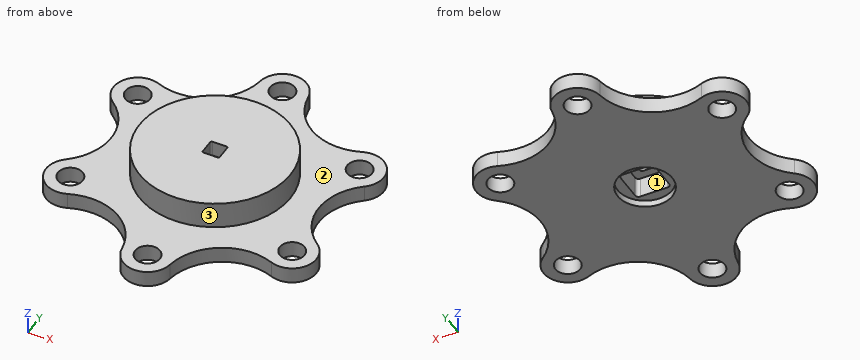
```python
from build123d import *

# Parameters (mm, degrees)
SKETCH1_R           = 2.3
BOSS_EXTRUDE1_DEPTH = 3
SKETCH2_R           = 14
BOSS_EXTRUDE2_DEPTH = 5
CUT_EXTRUDE1_REACH  = 40.688
SKETCH3_W           = 3.175
SKETCH3_H           = 3.175
SKETCH3_3_R         = 5.08
SKETCH3_3_W         = 6.35
SKETCH3_3_H         = 6.35
SKETCH3_3_W_2       = 3.175
SKETCH3_3_H_2       = 3.175
CUT_EXTRUDE2_DEPTH  = 1.27
CUT_EXTRUDE3_START  = -1.27
SKETCH3_4_W         = 6.35
SKETCH3_4_H         = 6.35
SKETCH3_4_W_2       = 3.175
SKETCH3_4_H_2       = 3.175
CUT_EXTRUDE3_DEPTH  = 3.81
FILLET1_R           = 0.254
FILLET2_R           = 0.635


with BuildPart() as part:
    # Sketch1 → Boss-Extrude1 (new body)
    with BuildSketch(Plane.XY):
        with BuildLine():
            ThreePointArc((4.456432387, 24.437168219), (-4.5e-08, 28.3125), (-4.456432399, 24.43716813))
            ThreePointArc((-4.456432399, 24.43716813), (-9.656250022, 16.725115598), (-18.934992245, 16.077967752))
            ThreePointArc((-18.934992245, 16.077967752), (-24.519343502, 14.156251286), (-23.391426978, 8.359202257))
            ThreePointArc((-23.391426978, 8.359202257), (-19.3125, 3.465e-06), (-23.391421517, -8.359197993))
            ThreePointArc((-23.391421517, -8.359197993), (-24.519344633, -14.156249327), (-18.934990017, -16.077966851))
            ThreePointArc((-18.934990017, -16.077966851), (-9.65625113, -16.725114958), (-4.456433088, -24.437163215))
            ThreePointArc((-4.456433088, -24.437163215), (-2.557e-06, -28.3125), (4.456432378, -24.437168281))
            ThreePointArc((4.456432378, -24.437168281), (9.656248045, -16.725116739), (18.934988153, -16.077966097))
            ThreePointArc((18.934988153, -16.077966097), (24.519343112, -14.156251962), (23.391424728, -8.3592005))
            ThreePointArc((23.391424728, -8.3592005), (19.3125, 1.013e-06), (23.391426325, 8.359201747))
            ThreePointArc((23.391426325, 8.359201747), (24.519343744, 14.156250867), (18.934992375, 16.077967805))
            ThreePointArc((18.934992375, 16.077967805), (9.656250044, 16.725115585), (4.456432387, 24.437168219))
        make_face()
        with Locations((0, 23.8125)):
            Circle(SKETCH1_R, mode=Mode.SUBTRACT)
        with Locations((20.622229928, 11.90625)):
            Circle(SKETCH1_R, mode=Mode.SUBTRACT)
        with Locations((-20.622229928, 11.90625)):
            Circle(SKETCH1_R, mode=Mode.SUBTRACT)
        with Locations((20.622229928, -11.90625)):
            Circle(SKETCH1_R, mode=Mode.SUBTRACT)
        with Locations((-20.622229928, -11.90625)):
            Circle(SKETCH1_R, mode=Mode.SUBTRACT)
        with Locations((0, -23.8125)):
            Circle(SKETCH1_R, mode=Mode.SUBTRACT)
    extrude(amount=BOSS_EXTRUDE1_DEPTH)

    # Sketch2 → Boss-Extrude2 (add)
    with BuildSketch(Plane.XY.offset(3)):
        Circle(SKETCH2_R)
    extrude(amount=BOSS_EXTRUDE2_DEPTH)

    # Sketch3 → Cut-Extrude1 (cut, up to next)
    with BuildSketch(Plane(origin=(0, 0, 0), x_dir=(-1, 0, 0), z_dir=(0, 0, -1)), mode=Mode.PRIVATE) as cut_extrude1_sk1:
        Rectangle(SKETCH3_W, SKETCH3_H)
    cut_extrude1_tool1 = extrude(cut_extrude1_sk1.sketch, amount=-CUT_EXTRUDE1_REACH, mode=Mode.PRIVATE) & part.part
    add(cut_extrude1_tool1.solids().sort_by_distance((0, 0, 0))[0], mode=Mode.SUBTRACT)

    # Sketch3<3> → Cut-Extrude2 (cut)
    # profile 1 of 3: a face of its own
    with BuildSketch(Plane(origin=(0, 0, 0), x_dir=(-1, 0, 0), z_dir=(0, 0, -1))):
        Circle(SKETCH3_3_R)
        Rectangle(SKETCH3_3_W, SKETCH3_3_H, mode=Mode.SUBTRACT)
    # profile 2 of 3: a face of its own
    with BuildSketch(Plane(origin=(0, 0, 0), x_dir=(-1, 0, 0), z_dir=(0, 0, -1))):
        Rectangle(SKETCH3_3_W, SKETCH3_3_H)
        Rectangle(SKETCH3_3_W_2, SKETCH3_3_H_2, mode=Mode.SUBTRACT)
    # profile 3 of 3: a face of its own
    with BuildSketch(Plane(origin=(0, 0, 0), x_dir=(-1, 0, 0), z_dir=(0, 0, -1))):
        Rectangle(SKETCH3_3_W_2, SKETCH3_3_H_2)
    extrude(amount=-CUT_EXTRUDE2_DEPTH, mode=Mode.SUBTRACT)

    # Sketch3<4> → Cut-Extrude3 (cut)
    with BuildSketch(Plane(origin=(0, 0, 0), x_dir=(-1, 0, 0), z_dir=(0, 0, -1)).offset(CUT_EXTRUDE3_START)):
        Rectangle(SKETCH3_4_W, SKETCH3_4_H)
        Rectangle(SKETCH3_4_W_2, SKETCH3_4_H_2, mode=Mode.SUBTRACT)
    extrude(amount=-CUT_EXTRUDE3_DEPTH, mode=Mode.SUBTRACT)

    # Fillet1
    fillet1_edges = [part.edges().sort_by_distance(p)[0] for p in [
        (-1.5875, -1.5875, 6.54),
        (1.5875, -1.5875, 6.54),
        (1.5875, 1.5875, 6.54),
        (-1.5875, 1.5875, 6.54),
    ]]
    fillet(fillet1_edges, radius=FILLET1_R)

    # Fillet2
    fillet2_edges = [part.edges().sort_by_distance(p)[0] for p in [
        (3.175, -3.175, 3.175),
        (3.175, 3.175, 3.175),
        (-3.175, 3.175, 3.175),
        (-3.175, -3.175, 3.175),
    ]]
    fillet(fillet2_edges, radius=FILLET2_R)


solid = part.part
```
CAD build for the part. Positions are in the model's coordinates, mm. Face numbers are marked on the shaded views. Coordinates: 2 decimals unless noted, no trailing zeros. Order: outer loops, then holes, each group sorted by start corner. A loop starts at its lowest first (then second) coordinate and runs counter-clockwise, first axis right, second up. Notation, with made-up numbers: M -38.75,57.5 L 2.25,57.5 A29 cw 2.25,86.5 Z; hole C 52,57 d3. An arc over 180 degrees is marked long. Write each question's results on one line, items separated by ' | '. Start each with the question number.
Q1. Cut at C-C (y = 0). List the corners of the cut face in (x, z) (1 decimal).
Q2. Cut at D-D (x = -9). List the corners of the cut face in (y, z), then the cut area to 3 significant figures.
Q3. Pull direction Y, two halves, no side cores. Call the marked faces 1, 2 and 3: +Y half, -Y half, draft (parallel to the pull), parting line (faces both ways), or undercut.
Q4. Flat gauge pins, fed straight in: P1, Ø2, axis at x = -0.5, z = 7, coming from the +Y side; P2, Ø1, axis at x = 4.5, z = 3, coming from the +Y side; P3, Ø4, axis at x = 10, y = -18.5, coming from the +Z side. Where does each tip first touch, or does it go through?
Q5. Cut at B-B (z = 3.75). List the corners of the cut face in (x, y) (3 decimals).
Q6. Drill centre lines: probe 1 along Y at (x, z) = (0, 0.6); probe 2 along X at (y, z) = (0.5, 2) (3 decimals); probe 3 along X at (y, z) = (-13, 2). Where is each one in solid material? Low to high. Write a range as from..to.
Q7. Cut at A-A (x = 0). List the corners of the cut face in (y, z) (1 decimal).
Found:
1) outline: M -19.3,0 L -5.1,0 L -5.1,1.3 L -3.2,1.3 L -3.2,5.1 L -1.6,5.1 L -1.6,8 L -14,8 L -14,3 L -19.3,3 Z; M 1.6,5.1 L 3.2,5.1 L 3.2,1.3 L 5.1,1.3 L 5.1,0 L 19.3,0 L 19.3,3 L 14,3 L 14,8 L 1.6,8 Z
2) outline: M -17.14,0 L 17.14,0 L 17.14,3 L 10.72,3 L 10.72,8 L -10.72,8 L -10.72,3 L -17.14,3 Z | area: 210 mm²
3) face 1: undercut | face 2: draft | face 3: parting line
4) P1: y = 14 | P2: y = 25.87 | P3: z = 3
5) outline: C 0,0 d28; hole M -3.175,-2.54 A0.635 ccw -2.54,-3.175 L 2.54,-3.175 A0.635 ccw 3.175,-2.54 L 3.175,2.54 A0.635 ccw 2.54,3.175 L -2.54,3.175 A0.635 ccw -3.175,2.54 Z
6) probe 1: -28.31..-26.11, -21.51..-5.08, 5.08..21.51, 26.11..28.31 | probe 2: -19.324..-3.175, 3.175..19.324 | probe 3: -24.99..-22.65, -18.6..18.6, 22.65..24.99
7) outline: M -28.3,0 L -26.1,0 L -26.1,3 L -28.3,3 Z; M -21.5,0 L -5.1,0 L -5.1,1.3 L -3.2,1.3 L -3.2,5.1 L -1.6,5.1 L -1.6,8 L -14,8 L -14,3 L -21.5,3 Z; M 1.6,5.1 L 3.2,5.1 L 3.2,1.3 L 5.1,1.3 L 5.1,0 L 21.5,0 L 21.5,3 L 14,3 L 14,8 L 1.6,8 Z; M 26.1,0 L 28.3,0 L 28.3,3 L 26.1,3 Z
